```python
from build123d import *

# Parameters (mm, degrees)
CROQUIS2_R                 = 3.5
SALIENTE_EXTRUIR1_DEPTH    = 20
CROQUIS3_R                 = 7.5
SALIENTE_EXTRUIR2_DEPTH    = 1
CROQUIS5_R                 = 9
SALIENTE_EXTRUIR3_DEPTH    = 4
CORTAR_EXTRUIR1_DEPTH      = 5
CORTAR_EXTRUIR1_DEPTH_BACK = 5
CROQUIS6_R                 = 4.25
CROQUIS7_R                 = 0.75
CORTAR_EXTRUIR2_DEPTH      = 5


with BuildPart() as part:
    # Croquis2 → Saliente-Extruir1 (new body)
    with BuildSketch(Plane(origin=(0, 0, 0), x_dir=(1, 0, 0), z_dir=(0, 1, 0))):
        with Locations(Location((0, 0, 0), (0, 0, 270))):
            Circle(CROQUIS2_R)
    extrude(amount=SALIENTE_EXTRUIR1_DEPTH)

    # Croquis3 → Saliente-Extruir2 (add)
    with BuildSketch(Plane(origin=(0, 20, 0), x_dir=(1, 0, 0), z_dir=(0, 1, 0))):
        with Locations(Location((0, 0, 0), (0, 0, 270))):
            Circle(CROQUIS3_R)
    extrude(amount=SALIENTE_EXTRUIR2_DEPTH)

    # Croquis5 → Saliente-Extruir3 (add)
    with BuildSketch(Plane(origin=(0, 21, 0), x_dir=(1, 0, 0), z_dir=(0, 1, 0))):
        with Locations(Location((0, 0, 0), (0, 0, 270))):
            Circle(CROQUIS5_R)
    extrude(amount=SALIENTE_EXTRUIR3_DEPTH)

    # Croquis6 → Cortar-Extruir1 (cut, two sides: drawn at the far end of the back side and taken through both)
    with BuildSketch(Plane.XY.offset(-CORTAR_EXTRUIR1_DEPTH_BACK)):
        with Locations((0, 25)):
            Circle(CROQUIS6_R)
    extrude(amount=CORTAR_EXTRUIR1_DEPTH + CORTAR_EXTRUIR1_DEPTH_BACK, mode=Mode.SUBTRACT)

    # Croquis7 → Cortar-Extruir2 (cut)
    with BuildSketch(Plane.XZ):
        with Locations(Location((0, 0, 0), (0, 0, 270))):
            Circle(CROQUIS7_R)
    extrude(amount=-CORTAR_EXTRUIR2_DEPTH, mode=Mode.SUBTRACT)


solid = part.part
```
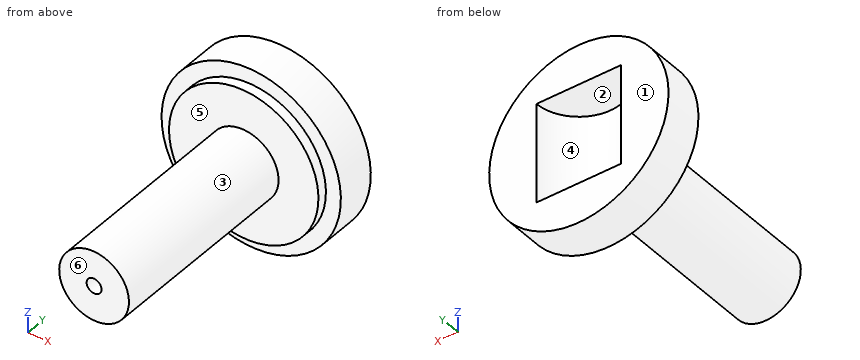
CAD build for the part. Positions are in the model's coordinates, mm. Face numbers are marked on the shaded views. A direction names the side the tool comes from. Coordinates: 2 decimals unless noted, no trailing zeros. Order: outer loops, then holes, each group sorted by start corner. A loop starts at its lowest first (then second) coordinate and runs counter-clockwise, first axis right, second up.
(1) Drill centre lines: L1, parallel to X at y = 3.85, z = 0; L2, parallel to Y at x = 5, z = 5.25; L3, parallel to Z at x = 0.5, y = 4. Where is each one in solid material? Low to high.
Solution:
L1: x = -3.5 to -0.75, 0.75 to 3.5
L2: y = 20 to 25
L3: z = -3.46 to -0.56, 0.56 to 3.46
(2) Saw through at D-D, the plane y = 13. Write the cut outline in (x, z).
Solution:
outline: circle Ø7 at (0, 0)
(3) Saw through at B-B, the plane x = 0. Write the cut outline in (y, z), and give its area (3 significant figures).
Solution:
outline: (0, -3.5) - (20, -3.5) - (20, -7.5) - (21, -7.5) - (21, -9) - (25, -9) - (25, -5) - (20.75, -5) - (20.75, 5) - (25, 5) - (25, 9) - (21, 9) - (21, 7.5) - (20, 7.5) - (20, 3.5) - (0, 3.5) - (0, 0.75) - (5, 0.75) - (5, -0.75) - (0, -0.75) - close
area: 177 mm2
(4) Saw through at C-C, the plane y = 21.75. Write the cut outline in (x, z), and give its area (3 significant figures).
Solution:
outline: circle Ø18 at (0, 0); hole (-2.74, -5) - (2.74, -5) - (2.74, 5) - (-2.74, 5) - close
area: 200 mm2
(5) Saw through at A-A, the plane z = 0. Write the cut outline in (x, y).
Solution:
outline: (-9, 21) - (-7.5, 21) - (-7.5, 20) - (-3.5, 20) - (-3.5, 0) - (-0.75, 0) - (-0.75, 5) - (0.75, 5) - (0.75, 0) - (3.5, 0) - (3.5, 20) - (7.5, 20) - (7.5, 21) - (9, 21) - (9, 25) - (4.25, 25) arc R4.25 cw to (-4.25, 25) - (-9, 25) - close
(6) Mould opens along Z. For the marked faces 1, 2 and 3 say: released by +Z, released by -Z, zero draft, split by the parting line, or undercut.
Solution:
face 1: zero draft
face 2: undercut
face 3: split by the parting line
(7) Pin check, flat tips, straight feed: pin 1 Ø5 at (y, z) = (3.5, -1) entering from -X; pin 2 Ø4 at (y, z) = (8, -6) entering from -X; pin 3 Ø1.3 at (x, y) = (-2, 23) entering from +Z; pin 4 Ø8 at (x, y) = (-5.5, 15.5) entering from +Z. Stop position of each tip, or through.
Solution:
pin 1: stops at x = -3.5
pin 2: passes through
pin 3: stops at z = 8.9
pin 4: stops at z = 3.16
(8) Which spindle directions (+Z, -Z, +X, -X, +Y, -Y) get a long thin tool onto all of the face, cutting with end or side? Do the marked faces 4, 5 and 6. Say none if no direction does.
Solution:
face 4: +Y
face 5: -Y
face 6: +Z, -Z, +X, -X, -Y
